For this review, take the finished solid that the model builds, in its own axes (mm). Face numbers are marked on the shaded views. A direction names the side the tool comes from. Coordinates: 2 decimals unless noted, no trailing zeros. Write each loop counter-clockwise with the first axis right and the second up, starting at its lowest first coordinate (ties: lowest second). Pieces come first, ordered by that corner, then holes. Notation, with made-up numbers: M -18.75,28.25 L 24.25,28.25 A29 ccw 24.25,55.25 Z; hole C 59.25,-37 d5. An arc over 180 degrees is marked long. Return JSON: item names as keys, results as strings.
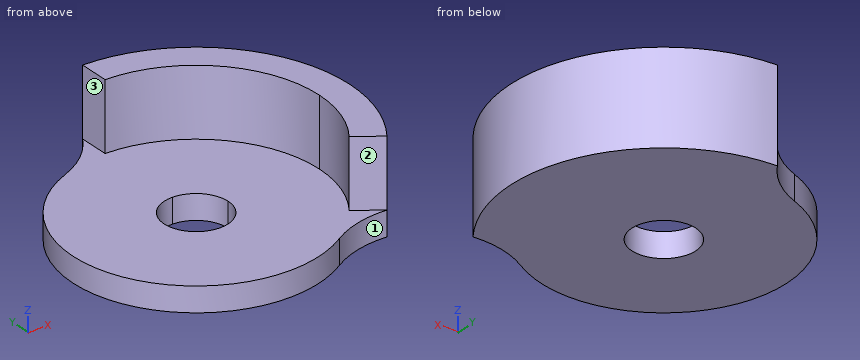
```python
from build123d import *

# Parameters (mm, degrees)
F1_DEPTH    = 1.27
F2_DEPTH    = 4.7625
F3_T1_DEPTH = 1.27


# Not quite as in the source:
# - a fillet or chamfer that OpenCascade refuses, or shapes differently, is made with other operations: its cross-section is extruded or revolved along the edge and cut away or added
# - a feature names something its author has since deleted; it is built from what else it names


with BuildPart() as f1:
    # F0 (on Top) → F1 (new body)
    with BuildSketch(Plane.XY):
        with BuildLine():
            ThreePointArc((5.2108397025, -3.6290011842), (6.0585201209, -1.9017975562), (6.35, 0))
            ThreePointArc((6.35, 0), (4.4901280605, 4.4901280605), (0, 6.35))
            Line((0, 6.35), (0, 5.1572436072))
            ThreePointArc((0, 5.1572436072), (3.6467219269, 3.6467219269), (5.1572436072, 0))
            ThreePointArc((5.1572436072, 0), (4.9205140413, -1.5445721714), (4.2320582273, -2.9473453792))
            Line((4.2320582273, -2.9473453792), (5.2108397025, -3.6290011842))
        make_face()
        with BuildLine():
            ThreePointArc((0, 6.35), (4.4901280605, 4.4901280605), (6.35, 0))
            ThreePointArc((6.35, 0), (6.0585201209, -1.9017975562), (5.2108397025, -3.6290011842))
            Line((5.2108397025, -3.6290011842), (6.4969090936, -4.5246624615))
            ThreePointArc((6.4969090936, -4.5246624615), (7.5538025952, -2.3711736577), (7.9172216188, 0))
            ThreePointArc((7.9172216188, 0), (5.5983210948, 5.5983210948), (0, 7.9172216188))
            Line((0, 7.9172216188), (0, 6.35))
        make_face()
        with BuildLine():
            Line((0, 5.1572436072), (0, 6.35))
            ThreePointArc((0, 6.35), (-5.6287946099, -2.939246713), (5.2108397025, -3.6290011842))
            Line((5.2108397025, -3.6290011842), (4.2320582273, -2.9473453792))
            ThreePointArc((4.2320582273, -2.9473453792), (-4.571506302, -2.3871513891), (0, 5.1572436072))
        make_face()
        with BuildLine():
            Line((0, 1.651), (0, 5.1572436072))
            ThreePointArc((0, 5.1572436072), (-4.571506302, -2.3871513891), (4.2320582273, -2.9473453792))
            Line((4.2320582273, -2.9473453792), (1.3548183226, -0.9435403079))
            ThreePointArc((1.3548183226, -0.9435403079), (-1.4634865986, -0.7642041454), (0, 1.651))
        make_face()
        with BuildLine():
            ThreePointArc((5.1572436072, 0), (3.6467219269, 3.6467219269), (0, 5.1572436072))
            Line((0, 5.1572436072), (0, 1.651))
            ThreePointArc((0, 1.651), (1.1674332957, 1.1674332957), (1.651, 0))
            ThreePointArc((1.651, 0), (1.5752152314, -0.4944673646), (1.3548183226, -0.9435403079))
            Line((1.3548183226, -0.9435403079), (4.2320582273, -2.9473453792))
            ThreePointArc((4.2320582273, -2.9473453792), (4.9205140413, -1.5445721714), (5.1572436072, 0))
        make_face()
    extrude(amount=F1_DEPTH)

    # F0 (on Top) → F2 (join)
    with BuildSketch(Plane.XY):
        with BuildLine():
            ThreePointArc((0, 6.35), (4.4901280605, 4.4901280605), (6.35, 0))
            ThreePointArc((6.35, 0), (6.0585201209, -1.9017975562), (5.2108397025, -3.6290011842))
            Line((5.2108397025, -3.6290011842), (6.4969090936, -4.5246624615))
            ThreePointArc((6.4969090936, -4.5246624615), (7.5538025952, -2.3711736577), (7.9172216188, 0))
            ThreePointArc((7.9172216188, 0), (5.5983210948, 5.5983210948), (0, 7.9172216188))
            Line((0, 7.9172216188), (0, 6.35))
        make_face()
    extrude(amount=F2_DEPTH)

    # F3: fillet of radius 5.08 on 2 edges, made by hand

    # F3_s2 → F3_t1 (join)
    with BuildSketch(Plane.XY):
        with BuildLine():
            ThreePointArc((0, 7.9172216188), (-1.0395816291, 6.7062044575), (-2.4036069424, 5.8775142421))
            ThreePointArc((-2.4036069424, 5.8775142421), (-1.2248029561, 6.2307590002), (0, 6.35))
            Line((0, 6.35), (0, 7.9172216188))
        make_face()
        with BuildLine():
            ThreePointArc((6.4969090936, -4.5246624615), (4.9090257444, -4.6856562433), (3.4494633266, -5.3313884456))
            ThreePointArc((3.4494633266, -5.3313884456), (4.4130196845, -4.5659344349), (5.2108397025, -3.6290011842))
            Line((5.2108397025, -3.6290011842), (6.4969090936, -4.5246624615))
        make_face()
    extrude(amount=F3_T1_DEPTH)


solid = f1.part
```
1. We need section B-B (x = -1.25). State the section outline as (y, z) points.
Checks:
{"outline": "M -6.23,0 L -1.08,0 L -1.08,1.27 L -6.23,1.27 Z; M 1.08,0 L 6.54,0 L 6.54,1.27 L 1.08,1.27 Z"}
2. We need section D-D (z = 3.9). State the section outline as (x, y) points, plus the area to 3 significant figures.
Checks:
{"outline": "M 0,6.35 A6.35 cw 5.21,-3.63 L 6.5,-4.52 A7.92 ccw 0,7.92 Z", "area": "24.4 mm2"}
3. We need section A-A (z = 0.75). State the section outline as (x, y) points.
Checks:
{"outline": "M -2.4,5.88 A6.35 ccw long 3.45,-5.33 A5.08 cw 6.5,-4.52 A7.92 ccw 0,7.92 A5.08 cw Z; hole C 0,0 d3.3"}
4. Wall thickness on L1, parallel to Z at x = 4, y = 4; L2, parallel to Y at x = 4.25, z = 1.45; L3, parallel to Y at x = 3, z = 0.3: over which ranges is each line inside the solid? List them lowest first. Write a range as from..to.
Checks:
{"L1": "0..1.27", "L2": "4.72..6.68", "L3": "-5.6..7.33"}
5. For the marked faces 1, 2 and 3, list the 3-axis set-ups (+Z, -Z, +X, -X, +Y, -Y) from which the entire face can be reached by the end or side of a thin tool; tool diameter is ignored.
Checks:
{"face 1": "+Z, -Z, -Y", "face 2": "+Z, -X, -Y", "face 3": "+Z, -X, +Y, -Y"}
6. Clearance check with flat-ended pins moving along their axes: pin 1 Ø2 at (y, z) = (-5, 4) entering from +X; pin 2 Ø0.8 at (y, z) = (7, 3) entering from -X; pin 3 Ø6.5 at (x, y) = (0, 0.5) entering from +Z. State where each tip first meets the part, or that it passes through.
Checks:
{"pin 1": "x = 6.83", "pin 2": "x = 0", "pin 3": "z = 1.27"}
7. We need section C-C (y = 0.75). State the section outline as (x, z) points, plus the area to 3 significant figures.
Checks:
{"outline": "M -6.31,0 L -1.47,0 L -1.47,1.27 L -6.31,1.27 Z; M 1.47,0 L 7.88,0 L 7.88,4.76 L 6.31,4.76 L 6.31,1.27 L 1.47,1.27 Z", "area": "19.8 mm2"}
